from build123d import *

# Parameters (mm, degrees)
BOSS_EXTRUDE1_DEPTH = 3
BOSS_EXTRUDE2_DEPTH = 50
CUT_EXTRUDE1_REACH  = 51
CUT_EXTRUDE2_REACH  = 5
CUT_EXTRUDE3_REACH  = 51
SKETCH7_W           = 7
SKETCH7_H           = 12
CUT_EXTRUDE5_REACH  = 51
SKETCH8_W           = 7
SKETCH8_H           = 12
CUT_EXTRUDE7_REACH  = 5
SKETCH1_R           = 1.75


with BuildPart() as part:
    # Sketch2 → Boss-Extrude1 (new body)
    with BuildSketch(Plane(origin=(0, 0, 0), x_dir=(1, 0, 0), z_dir=(0, 1, 0))):
        Polygon((-52.5, 25), (52.5, 25), (76.5, 25), (79.5, 25), (79.5, -25), (76.5, -25), (52.5, -25), (-52.5, -25), (-76.5, -25), (-79.5, -25), (-79.5, 25), (-76.5, 25), align=None)
    extrude(amount=BOSS_EXTRUDE1_DEPTH)

    # Sketch4 → Boss-Extrude2 (add)
    with BuildSketch(Plane(origin=(0, 0, -25), x_dir=(-1, 0, 0), z_dir=(0, 0, -1))):
        Polygon((79.5, 0), (79.5, -46), (53.5, -46), (53.5, -43), (76.5, -43), (76.5, 0), align=None)
    boss_extrude2 = extrude(amount=-BOSS_EXTRUDE2_DEPTH)

    # Mirror1: Boss-Extrude2 across plane
    add(boss_extrude2.mirror(Plane(origin=(0, 0, 0), x_dir=(0, 0, 1), z_dir=(1, 0, 0))))

    # Sketch5 → Cut-Extrude1 (cut, up to next)
    with BuildSketch(Plane.XZ.offset(46), mode=Mode.PRIVATE) as cut_extrude1_sk1:
        with BuildLine():
            Line((-53.5, -2.375), (-60.5, -2.375))
            ThreePointArc((-60.5, -2.375), (-64.625, -6.5), (-60.5, -10.625))
            Line((-60.5, -10.625), (-53.5, -10.625))
            Line((-53.5, -10.625), (-53.5, -2.375))
        make_face()
    cut_extrude1_tool1 = extrude(cut_extrude1_sk1.sketch, amount=-CUT_EXTRUDE1_REACH, mode=Mode.PRIVATE) & part.part
    add(cut_extrude1_tool1.solids().sort_by_distance((-58.661274, -46, -6.5))[0], mode=Mode.SUBTRACT)

    # Sketch6 → Cut-Extrude2 (cut, up to next)
    with BuildSketch(Plane.XZ, mode=Mode.PRIVATE) as cut_extrude2_sk1:
        with BuildLine():
            Line((41.5, -2.375), (60.5, -2.375))
            ThreePointArc((60.5, -2.375), (64.625, -6.5), (60.5, -10.625))
            Line((60.5, -10.625), (41.5, -10.625))
            ThreePointArc((41.5, -10.625), (37.375, -6.5), (41.5, -2.375))
        make_face()
    cut_extrude2_tool1 = extrude(cut_extrude2_sk1.sketch, amount=-CUT_EXTRUDE2_REACH, mode=Mode.PRIVATE) & part.part
    add(cut_extrude2_tool1.solids().sort_by_distance((51, 0, -6.5))[0], mode=Mode.SUBTRACT)

    # Sketch7 → Cut-Extrude3 (cut, up to next)
    with BuildSketch(Plane.XZ.offset(46), mode=Mode.PRIVATE) as cut_extrude3_sk1:
        with Locations((70.5, 5)):
            Rectangle(SKETCH7_W, SKETCH7_H)
    cut_extrude3_tool1 = extrude(cut_extrude3_sk1.sketch, amount=-CUT_EXTRUDE3_REACH, mode=Mode.PRIVATE) & part.part
    add(cut_extrude3_tool1.solids().sort_by_distance((70.5, -46, 5))[0], mode=Mode.SUBTRACT)

    # Sketch8 → Cut-Extrude5 (cut, up to next)
    with BuildSketch(Plane(origin=(0, 3, 0), x_dir=(1, 0, 0), z_dir=(0, 1, 0)), mode=Mode.PRIVATE) as cut_extrude5_sk1:
        with Locations((-70.5, -5)):
            Rectangle(SKETCH8_W, SKETCH8_H)
    cut_extrude5_tool1 = extrude(cut_extrude5_sk1.sketch, amount=-CUT_EXTRUDE5_REACH, mode=Mode.PRIVATE) & part.part
    add(cut_extrude5_tool1.solids().sort_by_distance((-70.5, 3, 5))[0], mode=Mode.SUBTRACT)

    # Sketch1 → Cut-Extrude7 (cut, up to next)
    with BuildSketch(Plane(origin=(0, 0, 0), x_dir=(1, 0, 0), z_dir=(0, 1, 0)), mode=Mode.PRIVATE) as cut_extrude7_sk1:
        with Locations((-31.5, 20.5)):
            Circle(SKETCH1_R)
    cut_extrude7_tool1 = extrude(cut_extrude7_sk1.sketch, amount=CUT_EXTRUDE7_REACH, mode=Mode.PRIVATE) & part.part
    add(cut_extrude7_tool1.solids().sort_by_distance((-31.5, 0, -20.5))[0], mode=Mode.SUBTRACT)
    # Sketch1 → Cut-Extrude7 (cut, up to next)
    with BuildSketch(Plane(origin=(0, 0, 0), x_dir=(1, 0, 0), z_dir=(0, 1, 0)), mode=Mode.PRIVATE) as cut_extrude7_sk2:
        with Locations((-31.5, -20.5)):
            Circle(SKETCH1_R)
    cut_extrude7_tool2 = extrude(cut_extrude7_sk2.sketch, amount=CUT_EXTRUDE7_REACH, mode=Mode.PRIVATE) & part.part
    add(cut_extrude7_tool2.solids().sort_by_distance((-31.5, 0, 20.5))[0], mode=Mode.SUBTRACT)
    # Sketch1 → Cut-Extrude7 (cut, up to next)
    with BuildSketch(Plane(origin=(0, 0, 0), x_dir=(1, 0, 0), z_dir=(0, 1, 0)), mode=Mode.PRIVATE) as cut_extrude7_sk3:
        with Locations((31.5, -20.5)):
            Circle(SKETCH1_R)
    cut_extrude7_tool3 = extrude(cut_extrude7_sk3.sketch, amount=CUT_EXTRUDE7_REACH, mode=Mode.PRIVATE) & part.part
    add(cut_extrude7_tool3.solids().sort_by_distance((31.5, 0, 20.5))[0], mode=Mode.SUBTRACT)
    # Sketch1 → Cut-Extrude7 (cut, up to next)
    with BuildSketch(Plane(origin=(0, 0, 0), x_dir=(1, 0, 0), z_dir=(0, 1, 0)), mode=Mode.PRIVATE) as cut_extrude7_sk4:
        with Locations((31.5, 20.5)):
            Circle(SKETCH1_R)
    cut_extrude7_tool4 = extrude(cut_extrude7_sk4.sketch, amount=CUT_EXTRUDE7_REACH, mode=Mode.PRIVATE) & part.part
    add(cut_extrude7_tool4.solids().sort_by_distance((31.5, 0, -20.5))[0], mode=Mode.SUBTRACT)


solid = part.part
The listing builds one solid part. Answer for the finished solid, in the listing's coordinates (mm). A direction names the side the tool comes from. Coordinates: 2 decimals unless noted, no trailing zeros. Loops run counter-clockwise (first coordinate to the right, second up) from the corner with the lowest first, then second, coordinate; pieces in that order, holes last. Notation, with made-up numbers: M 13.25,-30 L 37.25,-30 A12 cw 37.25,-9 Z; hole C 22.5,69.25 d5. An arc over 180 degrees is marked long. Answer in a Markdown table with one row per item.
1) Find the intervals of material crossed by probe 1 along X at (y, z) = (1.05, -20.5); probe 2 along Z at (x, y) = (31.5, 1); probe 3 along X at (y, z) = (-23, -14), in increasing order.
Answers below:
| item | result |
|---|---|
| probe 1 | -79.5 to -33.25, -29.75 to 29.75, 33.25 to 79.5 |
| probe 2 | -25 to -22.25, -18.75 to 18.75, 22.25 to 25 |
| probe 3 | -79.5 to -76.5, 76.5 to 79.5 |
2) Given pin 1 (15 mm diameter, centred on x = 35.5, z = 7, fed in from -Y); pin 2 (3 mm diameter, centred on x = -31.5, z = 20.5, fed in from +Y), each flat-ended and moving along its own axis, determine where each tip first touches the part or whether it passes through.
Answers below:
| item | result |
|---|---|
| pin 1 | y = 0 |
| pin 2 | through |
3) Which of the six approach directions +Z, -Z, +X, -X, +Y, -Y give full straight-line access (tool end or side, diameter ignored) to faces 4 (the flat face through (-53.5, -45, -18)), 5 (the cylindrical face through (-64.624, -44.521, -6.409)), 6 (the cylindrical face through (64.624, 1.479, -6.409))?
Answers below:
| item | result |
|---|---|
| face 4 | +Z, -Z, -Y |
| face 5 | -Y |
| face 6 | +Y |
4) Determine the mould class of faces 1 (the flat face through (-65, -43, 0)), 2 (the flat face through (18, 0.4, 25)), 3 (the flat face through (-67, -46, 0)) for opening direction Y: released by +Y, released by -Y, zero draft, split by the parting line, or undercut.
Answers below:
| item | result |
|---|---|
| face 1 | undercut |
| face 2 | zero draft |
| face 3 | released by -Y |
5) Find section D-D (z = -6.5). Determine the outline of the cut face in (x, y) (3 decimals), then the cut area to 3 significant figures.
Answers below:
| item | result |
|---|---|
| outline | M -79.5,-46 L -64.625,-46 L -64.625,-43 L -76.5,-43 L -76.5,0 L 37.375,0 L 37.375,3 L -79.5,3 Z; M 53.5,-46 L 79.5,-46 L 79.5,3 L 64.625,3 L 64.625,0 L 76.5,0 L 76.5,-43 L 53.5,-43 Z |
| area | 776 mm^2 |
6) Find section C-C (x = 51.5). Determine the outline of the cut face in (y, z) (3 decimals).
Answers below:
| item | result |
|---|---|
| outline | M 0,-25 L 3,-25 L 3,-10.625 L 0,-10.625 Z; M 0,-2.375 L 3,-2.375 L 3,25 L 0,25 Z |
7) Find section A-A (y = -13.5). Determine the outline of the cut face in (x, z), then the cut area to 3 significant figures.
Answers below:
| item | result |
|---|---|
| outline | M -79.5,-25 L -76.5,-25 L -76.5,25 L -79.5,25 Z; M 76.5,-25 L 79.5,-25 L 79.5,25 L 76.5,25 Z |
| area | 300 mm^2 |
8) Find section B-B (z = 20.5). Determine the outline of the cut face in (x, y), then the cut area to 3 significant figures.
Answers below:
| item | result |
|---|---|
| outline | M -79.5,-46 L -53.5,-46 L -53.5,-43 L -76.5,-43 L -76.5,0 L -33.25,0 L -33.25,3 L -79.5,3 Z; M -29.75,0 L 29.75,0 L 29.75,3 L -29.75,3 Z; M 33.25,0 L 76.5,0 L 76.5,-43 L 53.5,-43 L 53.5,-46 L 79.5,-46 L 79.5,3 L 33.25,3 Z |
| area | 870 mm^2 |
